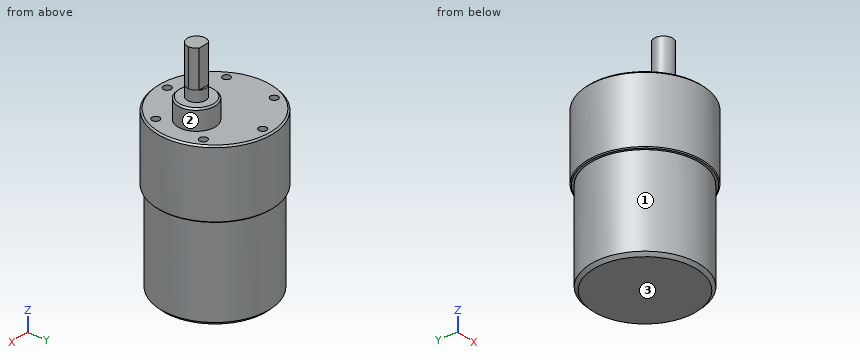
from build123d import *

# Parameters (mm, degrees)
SKETCH2_R                 = 17.5
BOSS_EXTRUDE1_DEPTH       = 30
SKETCH3_R                 = 18.5
BOSS_EXTRUDE2_DEPTH       = 22
M3X0_5_TAPPED_HOLE1_D     = 2.5
M3X0_5_TAPPED_HOLE1_DEPTH = 7.5
M3X0_5_TAPPED_HOLE1_TIP   = 0.751075774
SKETCH6_R                 = 6
BOSS_EXTRUDE3_DEPTH       = 6.5
SKETCH8_R                 = 3
BOSS_EXTRUDE4_DEPTH       = 3.5
BOSS_EXTRUDE5_DEPTH       = 12
CHAMFER1_SIZE             = 0.5
CHAMFER2_SIZE             = 0.5
CHAMFER3_SIZE             = 0.3
CHAMFER4_SIZE             = 1


with BuildPart() as part:
    # Sketch2 → Boss-Extrude1 (new body)
    with BuildSketch(Plane.XY):
        Circle(SKETCH2_R)
    extrude(amount=BOSS_EXTRUDE1_DEPTH)

    # Sketch3 → Boss-Extrude2 (add)
    with BuildSketch(Plane.XY.offset(30)):
        Circle(SKETCH3_R)
    extrude(amount=BOSS_EXTRUDE2_DEPTH)

    # M3x0.5 Tapped Hole1
    with Locations(Plane.XY.offset(52)):
        with Locations((13.423393759, -7.75), (13.423393759, 7.75), (0, 15.5), (-13.423393759, 7.75), (-13.423393759, -7.75), (0, -15.5)):
            Hole(M3X0_5_TAPPED_HOLE1_D / 2, depth=M3X0_5_TAPPED_HOLE1_DEPTH)
            with Locations((0, 0, -(M3X0_5_TAPPED_HOLE1_DEPTH + M3X0_5_TAPPED_HOLE1_TIP / 2))):  # 118° drill point
                Cone(0, M3X0_5_TAPPED_HOLE1_D / 2, M3X0_5_TAPPED_HOLE1_TIP, mode=Mode.SUBTRACT)

    # Sketch6 → Boss-Extrude3 (add)
    with BuildSketch(Plane.XY.offset(52)):
        with Locations(Location((7, 0, 0), (0, 0, 180))):
            Circle(SKETCH6_R)
    extrude(amount=BOSS_EXTRUDE3_DEPTH)

    # Sketch8 → Boss-Extrude4 (add)
    with BuildSketch(Plane.XY.offset(58.5)):
        with Locations((7, 0)):
            Circle(SKETCH8_R)
    extrude(amount=BOSS_EXTRUDE4_DEPTH)

    # Sketch9 → Boss-Extrude5 (add)
    with BuildSketch(Plane.XY.offset(62)):
        with BuildLine():
            Line((8.8, 2.4), (5.2, 2.4))
            ThreePointArc((5.2, 2.4), (5.658359214, -2.683281573), (10, 0))
            ThreePointArc((10, 0), (9.683281573, 1.341640786), (8.8, 2.4))
        make_face()
    extrude(amount=BOSS_EXTRUDE5_DEPTH)

    # Chamfer1
    chamfer1_edges = [part.edges().sort_by_distance(p)[0] for p in [
        (-18.5, 0, 52),
    ]]
    chamfer(chamfer1_edges, length=CHAMFER1_SIZE)

    # Chamfer2
    chamfer2_edges = [part.edges().sort_by_distance(p)[0] for p in [
        (13, 0, 58.5),
    ]]
    chamfer(chamfer2_edges, length=CHAMFER2_SIZE)

    # Chamfer3
    chamfer3_edges = [part.edges().sort_by_distance(p)[0] for p in [
        (-18.5, 0, 30),
    ]]
    chamfer(chamfer3_edges, length=CHAMFER3_SIZE)

    # Chamfer4
    chamfer4_edges = [part.edges().sort_by_distance(p)[0] for p in [
        (-17.5, 0, 0),
    ]]
    chamfer(chamfer4_edges, length=CHAMFER4_SIZE)


solid = part.part
Verification items for the finished model (mm, model axes). Face numbers are marked on the shaded views. A direction names the side the tool comes from. Round coordinates to 2 decimals unless told otherwise and drop trailing zeros. Loops run counter-clockwise (first coordinate to the right, second up) from the corner with the lowest first, then second, coordinate; pieces in that order, holes last. Notation, with made-up numbers: (3, -23.5) - (25, -23.5) arc R27 cw to (25, 13.5) - close; hole circle Ø9 at (77, 16.5). An arc over 180 degrees is marked (long way). Use a Markdown table: item, result. Add a question column.
1. Thickness scan on probe 1 along Y at (x, z) = (0, 50); probe 2 along Z at (x, y) = (-9, 1.5); probe 3 along X at (y, z) = (-7.75, 48.75). Record the ranges inside material, lowest first. Write a range as [from, to].
2. Section check A-A, the plane z = 37.5. Record the boundary of the cut face in (x, y).
3. Section check B-B, the plane z = 6. Record the boundary of the cut face in (x, y), plus the area to 3 significant figures.
4. Gauge pin test, flat ends, axial feed: pin 1 (5 mm diameter, centred on x = 3, y = 6, fed in from +Z); pin 2 (2 mm diameter, centred on x = -6, z = 9.5, fed in from -Y); pin 3 (6 mm diameter, centred on y = 9, z = 60, fed in from +X); pin 4 (4 mm diameter, centred on x = 0, y = 15.5, fed in from +Z). Record the tip position at first contact, or that the pin passes through.
5. Access from +Z, -Z, +X, -X, +Y, -Y to the whole of each face (thin tool, end or side, straight path). Record for the marked faces 1, 2 and 3.
Checks:
| question | item | result |
|---|---|---|
| 1 | probe 1 | y = [-18.5, -16.75], [-14.25, 14.25], [16.75, 18.5] |
| 1 | probe 2 | z = [0, 52] |
| 1 | probe 3 | x = [-16.8, -14.67], [-12.17, 12.17], [14.67, 16.8] |
| 2 | outline | circle Ø37 at (0, 0) |
| 3 | outline | circle Ø35 at (0, 0) |
| 3 | area | 962 mm^2 |
| 4 | pin 1 | stops at z = 58.5 |
| 4 | pin 2 | stops at y = -16.77 |
| 4 | pin 3 | passes through |
| 4 | pin 4 | stops at z = 52 |
| 5 | face 1 | -Z |
| 5 | face 2 | +Z |
| 5 | face 3 | -Z, +X, -X, +Y, -Y |
